Autodesk Inventor part; units mm, degrees
ref_plane "YZ Plane" through (0, 0, 0) normal (1, 0, 0) x (0, 1, 0)
ref_plane "XZ Plane" through (0, 0, 0) normal (0, 1, 0) x (-1, 0, 0)
ref_plane "XY Plane" through (0, 0, 0) normal (0, 0, 1) x (1, 0, 0)
sketch "Skizze1" plane through (0, 0, 0) normal (0, 0, 1) x (1, 0, 0)
  line L0 (7.75, -17.6806) -> (7.75, 17.6806)
  line L1 (-7.75, 17.6806) -> (-7.75, -17.6806)
  circle A0 centre (0, 0) radius 3.025
  arc A1 (-5.3363, -21.3526) -> (5.3363, -21.3526) centre (0, -9) ccw
  arc A2 (5.3363, -21.3526) -> (7.75, -17.6806) centre (3.75, -17.6806) ccw
  arc A3 (7.75, 17.6806) -> (5.3363, 21.3526) centre (3.75, 17.6806) ccw
  arc A4 (5.3363, 21.3526) -> (-5.3363, 21.3526) centre (0, 9) ccw
  arc A5 (-5.3363, 21.3526) -> (-7.75, 17.6806) centre (-3.75, 17.6806) ccw
  arc A6 (-7.75, -17.6806) -> (-5.3363, -21.3526) centre (-3.75, -17.6806) ccw
  circle A7 centre (-0.25, 17) radius 1.7
  circle A8 centre (-0.25, -7) radius 1.7
  line L2 (5.34, 14.1) -> (3.3, 14.1)
  line L3 (3.3, 14.1) -> (3.3, 17.74)
  line L4 (3.3, 17.74) -> (5.34, 17.74)
  line L5 (5.34, 17.74) -> (5.34, 14.1)
  line L6 (-3.8, 14.1) -> (-5.84, 14.1)
  line L7 (-5.84, 14.1) -> (-5.84, 17.74)
  line L8 (-5.84, 17.74) -> (-3.8, 17.74)
  line L9 (-3.8, 17.74) -> (-3.8, 14.1)
  circle A9 centre (-0.25, -15.278) radius 2.9
  point P0 (0, 0)
  point P1 (-17.1225, -5.975)
  point P2 (-17.1225, -12.025)
  point P3 (-17.1225, 6.3)
  point P4 (-17.1225, -14.3)
  point P5 (-17.1225, -17.7)
extrude "Extrusion1" add sketch "Skizze1" along normal blind 4 contours A2 A1 A6 L1 A5 A4 A3 L0 | A0 | A7 | A8 | L2 L3 L4 L5 | L6 L7 L8 L9 | A9
sketch "Skizze2" plane through (0, 0, 0) normal (0, 0, -1) x (-1, 0, 0)
  circle A0 centre (0, 0) radius 3.025
  arc A1 (-5.3363, -21.3526) -> (5.3363, -21.3526) centre (0, -9) ccw
  arc A2 (-7.75, -17.6806) -> (-5.3363, -21.3526) centre (-3.75, -17.6806) ccw
  line L0 (-7.75, -17.6806) -> (-7.75, 17.6806)
  arc A3 (-5.3363, 21.3526) -> (-7.75, 17.6806) centre (-3.75, 17.6806) ccw
  arc A4 (5.3363, 21.3526) -> (-5.3363, 21.3526) centre (0, 9) ccw
  arc A5 (7.75, 17.6806) -> (5.3363, 21.3526) centre (3.75, 17.6806) ccw
  line L1 (7.75, 17.6806) -> (7.75, -17.6806)
  arc A6 (5.3363, -21.3526) -> (7.75, -17.6806) centre (3.75, -17.6806) ccw
  circle A7 centre (0.25, 17) radius 1.7
  circle A8 centre (0.25, -7) radius 1.7
  line L2 (-5.34, 14.1) -> (-3.3, 14.1)
  line L3 (-3.3, 14.1) -> (-3.3, 17.74)
  line L4 (-3.3, 17.74) -> (-5.34, 17.74)
  line L5 (-5.34, 17.74) -> (-5.34, 14.1)
  line L6 (3.8, 14.1) -> (5.84, 14.1)
  line L7 (5.84, 14.1) -> (5.84, 17.74)
  line L8 (5.84, 17.74) -> (3.8, 17.74)
  line L9 (3.8, 17.74) -> (3.8, 14.1)
  circle A9 centre (0.25, -15.278) radius 2.9
  point P0 (0, 0)
extrude "Extrusion2" cut sketch "Skizze2" against normal blind 3.1 contours A0
sketch "Skizze3" plane through (0, 0, 0) normal (0, 0, -1) x (-1, 0, 0)
  circle A0 centre (0, 0) radius 3.025
  arc A1 (-5.3363, -21.3526) -> (5.3363, -21.3526) centre (0, -9) ccw
  arc A2 (-7.75, -17.6806) -> (-5.3363, -21.3526) centre (-3.75, -17.6806) ccw
  line L0 (-7.75, -17.6806) -> (-7.75, 17.6806)
  arc A3 (-5.3363, 21.3526) -> (-7.75, 17.6806) centre (-3.75, 17.6806) ccw
  arc A4 (5.3363, 21.3526) -> (-5.3363, 21.3526) centre (0, 9) ccw
  arc A5 (7.75, 17.6806) -> (5.3363, 21.3526) centre (3.75, 17.6806) ccw
  line L1 (7.75, 17.6806) -> (7.75, -17.6806)
  arc A6 (5.3363, -21.3526) -> (7.75, -17.6806) centre (3.75, -17.6806) ccw
  circle A7 centre (0.25, 17) radius 1.7
  circle A8 centre (0.25, -7) radius 1.7
  line L2 (-5.34, 14.1) -> (-3.3, 14.1)
  line L3 (-3.3, 14.1) -> (-3.3, 17.74)
  line L4 (-3.3, 17.74) -> (-5.34, 17.74)
  line L5 (-5.34, 17.74) -> (-5.34, 14.1)
  line L6 (3.8, 14.1) -> (5.84, 14.1)
  line L7 (5.84, 14.1) -> (5.84, 17.74)
  line L8 (5.84, 17.74) -> (3.8, 17.74)
  line L9 (3.8, 17.74) -> (3.8, 14.1)
  circle A9 centre (0.25, -15.278) radius 2.9
  point P0 (0, 0)
hole "Bohrung1" at (-0.25, 17, 0) at (-0.25, -7, 0) direction (0, 0, 1) diameter 5.6 depth 3.2 counterbore diameter 7.1 counterbore depth 1.2
sketch "Skizze4" plane through (0, 0, 4) normal (0, 0, 1) x (1, 0, 0)
  circle A0 centre (-0.25, 17) radius 3.55
  circle A1 centre (-0.25, -7) radius 3.55
  circle A2 centre (0, 0) radius 3.025
  arc A3 (5.3363, -21.3526) -> (7.75, -17.6806) centre (3.75, -17.6806) ccw
  arc A4 (-5.3363, -21.3526) -> (5.3363, -21.3526) centre (0, -9) ccw
  arc A5 (-7.75, -17.6806) -> (-5.3363, -21.3526) centre (-3.75, -17.6806) ccw
  line L0 (-7.75, 17.6806) -> (-7.75, -17.6806)
  arc A6 (-5.3363, 21.3526) -> (-7.75, 17.6806) centre (-3.75, 17.6806) ccw
  arc A7 (5.3363, 21.3526) -> (-5.3363, 21.3526) centre (0, 9) ccw
  arc A8 (7.75, 17.6806) -> (5.3363, 21.3526) centre (3.75, 17.6806) ccw
  line L1 (7.75, -17.6806) -> (7.75, 17.6806)
  circle A9 centre (12.6079, -10) radius 2.8
  circle A10 centre (12.6079, -10) radius 2.8
  line L2 (4.1087, 0) -> (7.1087, 0)
  line L3 (7.1087, 0) -> (2.8877, -6.1994)
  line L4 (2.8877, -6.1994) -> (-0.1123, -6.1994)
  line L5 (-0.1123, -6.1994) -> (4.1087, 0)
  line L6 (2.721, 6.1994) -> (5.721, 6.1994)
  line L7 (5.721, 6.1994) -> (-2.721, -6.1994)
  line L8 (-2.721, -6.1994) -> (-5.721, -6.1994)
  line L9 (-5.721, -6.1994) -> (2.721, 6.1994)
  line L10 (-2.8877, 6.1994) -> (0.1123, 6.1994)
  line L11 (0.1123, 6.1994) -> (-4.1087, 0)
  line L12 (-4.1087, 0) -> (-7.1087, 0)
  line L13 (-7.1087, 0) -> (-2.8877, 6.1994)
  line L14 (7.1087, 6.1994) -> (7.1087, -6.1994)
  line L15 (7.1087, -6.1994) -> (-7.1087, -6.1994)
  line L16 (-7.1087, -6.1994) -> (-7.1087, 6.1994)
  line L17 (-7.1087, 6.1994) -> (7.1087, 6.1994)
  point P0 (0, 0)
  point P1 (16.5579, -10)
  point P2 (16.5579, -10)
  point P3 (16.5579, -10)
  point P4 (50.5428, -9.282)
  point P5 (-4.221, -6.1994)
  point P6 (4.221, 6.1994)
  point P7 (-1.3877, 6.1994)
  point P8 (1.3877, -6.1994)
  dimension "d89" = 5.6
  dimension "d104" = 5.6
  dimension "d107" = 14.2174
  dimension "d108" = 12.3988
  dimension "d109" = 2.1563
  dimension "d110" = 2.1563
  dimension "d111" = 2.4798
  dimension "d112" = 2.4798
  dimension "d113" = 2.4798
  dimension "d114" = 6.1994
  dimension "d115" = 6.1994
  dimension "d116" = 6.1994
  dimension "d117" = 15.5
  dimension "d118" = 0.6413
move faces "Verschieben1" translate (0, 0, 0.5) faces at (-2.5833, -5.8935, 4)
extrude "Extrusion4" cut sketch "Skizze4" along normal mid plane 0.8 contours L8 L9 A2 L7 A1 | A1 L7 L8 | L3 L4 L5 A1 | A1 L5 L2 L3 | A2 L9 L7 | A2 L9 L6 L7 | L13 L10 L11 L12
extrude "Extrusion5" cut sketch "Skizze4" along normal through all contours L8 L9 A2 L7 A1 | A1 L7 L8 | L3 L4 L5 A1 | A1 L5 L2 L3 | A2 L9 L7 | A2 L9 L6 L7 | L13 L10 L11 L12
sketch "Skizze5" plane through (0, 0, 0) normal (0, 0, -1) x (-1, 0, 0)
  circle A0 centre (0.25, -15.278) radius 2.9
  point P0 (0, 0)
extrude "Extrusion6" cut sketch "Skizze5" against normal blind 1.4
chamfer "Fase2" distance 0.2 distance2 0.8 1 edges at (-0.25, -10.55, 0) measured on face at (6.175, 0, 0)
chamfer "Fase3" distance 2 distance2 0.4 1 edges at (-0.25, -9.8, 1.2) measured on face at (0.1992, -4.2363, 2.5333)
chamfer "Fase4" distance 2 distance2 0.4 1 edges at (-0.25, 14.2, 1.2) measured on face at (0.1992, 19.7637, 2.5333)
chamfer "Fase5" distance 0.2 distance2 0.8 1 edges at (-0.25, 13.45, 0) measured on face at (6.175, 0, 0)
chamfer "Fase6" distance 0.4 angle 45 8 edges at (-7.75, 0, 0) (-7.0925, -19.8777, 0) (0, -22.4559, 0) (7.0925, -19.8777, 0) (7.75, 0, 0) (7.0925, 19.8777, 0) (0, 22.4559, 0) (-7.0925, 19.8777, 0)
properties part number "Cover_Squared"
Geometry: final body of the model. Coordinates: model frame, mm. A direction names the side the tool comes from. Coordinates: 2 decimals unless noted, no trailing zeros. One line per item, written item: value. Start each with the question number.
1) Material intervals for L1, parallel to Y at x = -2.5, z = 2.6; L2, parallel to Y at x = 0, z = 2.2 (1 decimal); L3, parallel to X at y = -7, z = 1.15, sorted ascending. Write a range as from..to.
2) Pin query (flat end, axial travel): P1, Ø1.5, axis at x = -1, z = 3, coming from the +Y side; P2, Ø1.8, axis at x = 1.5, y = -1, coming from the -Z side; P3, Ø0.7, axis at x = 5, z = 4, coming from the -Y side; P4, Ø5.5, axis at x = 0, y = 0, coming from the +Z side. Return the tip coordinate at first contact, or that it passes through.
3) Reachability of faces 5 (the cylindrical face through (0.077, -22.456, 2.421)), 6 (the cylindrical face through (-1.316, 20.386, 1.003)), 7 (the flat face through (-4, -6.199, 4)) from +Z, -Z, +X, -X, +Y, -Y: full face, straight path, thin tool, end or side. Return the list, or none.
4) Draft query along Y for faces 1 (the cylindrical face through (0.1, -12.4, 0.7)), 2 (the cylindrical face through (7.075, 19.905, 2.421)), 3 (the flat face through (7.75, 0, 2)), 4 (the cylindrical face through (7.11, -19.85, 2.42)). Return one class per face: released by +Y, released by -Y, zero draft, split by the parting line, or undercut.
Evaluation:
1. L1: -22.22..-8.86, -5.14..-1.7, 1.7..15.14, 18.86..22.22
1. L2: -22.5..-10, -4..-3, 3..14, 20..22.5
1. L3: -7.75..-3.8, 3.3..7.75
2. P1: y = 22.45
2. P2: z = 3.1
2. P3: y = -21.63
2. P4: z = 4.5
3. face 5: +Z, -Z, -Y
3. face 6: -Z
3. face 7: +Z
4. face 1: undercut
4. face 2: released by +Y
4. face 3: zero draft
4. face 4: released by -Y
